Design review of the part built by this model. Coordinates are the model's own, in mm. Round coordinates to 2 decimals unless told otherwise and drop trailing zeros. Order: outer loops, then holes, each group sorted by start corner. A loop starts at its lowest first (then second) coordinate and runs counter-clockwise, first axis right, second up. Notation, with made-up numbers: M -17,42 L -13,42 A30 cw -13,67 Z; hole C -36.5,46 d1. An arc over 180 degrees is marked long. Write each question's results on one line, items separated by ' | '. Start each with the question number.
Item 1: Clearance check with a flat-ended pin moving along its axis: pin 1 (2 mm diameter, centred on x = 0, z = 0.5, fed in from -Y). State where the tip first meets the part, or that it passes through.
Item 2: Take a section at B-B, the plane y = 3.75. Write out the cut boundary in (x, z), plus the area to 3 significant figures.
Item 3: Take a section at A-A, the plane x = 0. Write out the cut boundary in (y, z).
Item 4: Take a section at C-C, the plane y = 2.25. Write out the cut boundary in (x, z), plus the area to 3 significant figures.
Item 5: Wall thickness on line 1 (Z direction, x = 0, y = 0.3); line 2 (X direction, y = 0.5, z = 0.25); line 3 (Z direction, x = 0.75, y = 2.5): over which ranges is each line inside the solid? List them lowest first. Write a range as [from, to].
Item 6: The part is to be moulded in two halves that separate along Z. For faces 1 (the flat face through (0, 0, 0.4)), 2 (the conical face through (1.198, 5.07, -0.377)), 3 (the flat face through (0.01, 1, 0.45)), say which applies: +Z half, -Z half, draft (parallel to the pull), parting line (faces both ways), or undercut.
```python
from build123d import *

# Parameters (mm, degrees)
IZIM1_R                     = 1.7
Y_KSEKLIK_EKSTR_ZYON1_DEPTH = 10
Y_KSEKLIK_EKSTR_ZYON1_TAPER = 5
IZIM2_R                     = 1.122825905
KES_EKSTR_ZYON1_DEPTH       = 10
KES_EKSTR_ZYON1_TAPER       = 4
IZIM3_R                     = 1.122825905
IZIM3_R_2                   = 0.19962026
IZIM3_R_3                   = 0.196792851
IZIM3_R_4                   = 0.203205658
IZIM3_R_5                   = 0.197119951
Y_KSEKLIK_EKSTR_ZYON3_DEPTH = 1
IZIM5_R                     = 0.197735833
IZIM5_R_2                   = 0.2
KES_EKSTR_ZYON2_DEPTH       = 1
IZIM6_R                     = 0.196695493
KES_EKSTR_ZYON3_DEPTH       = 1


with BuildPart() as part:
    # Çizim1 → Yükseklik-Ekstrüzyon1 (new body)
    with BuildSketch(Plane(origin=(0, 0, 0), x_dir=(1, 0, 0), z_dir=(0, 1, 0))):
        Circle(IZIM1_R)
    extrude(amount=Y_KSEKLIK_EKSTR_ZYON1_DEPTH, taper=Y_KSEKLIK_EKSTR_ZYON1_TAPER)

    # Çizim2 → Kes-Ekstrüzyon1 (cut)
    with BuildSketch(Plane.XZ):
        Circle(IZIM2_R)
    extrude(amount=-KES_EKSTR_ZYON1_DEPTH, taper=KES_EKSTR_ZYON1_TAPER, mode=Mode.SUBTRACT)

    # Çizim3 → Yükseklik-Ekstrüzyon3 (add)
    with BuildSketch(Plane(origin=(0, 0, 0), x_dir=(-1, 0, 0), z_dir=(0, -1, 0))):
        Circle(IZIM3_R)
        with Locations((-0.353553391, -0.353553391)):
            Circle(IZIM3_R_2, mode=Mode.SUBTRACT)
        with Locations((-0.353553391, 0.353553391)):
            Circle(IZIM3_R_3, mode=Mode.SUBTRACT)
        with Locations((0.353553391, 0.353553391)):
            Circle(IZIM3_R_4, mode=Mode.SUBTRACT)
        with Locations((0.353553391, -0.353553391)):
            Circle(IZIM3_R_5, mode=Mode.SUBTRACT)
    extrude(amount=-Y_KSEKLIK_EKSTR_ZYON3_DEPTH)

    # Çizim5 → Kes-Ekstrüzyon2 (cut)
    with BuildSketch(Plane.XZ):
        with Locations((0.8, 0)):
            Circle(IZIM5_R)
        with Locations((-0.8, 0)):
            Circle(IZIM5_R_2)
        with Locations((0, -0.8)):
            Circle(IZIM5_R)
        with Locations((0, 0.8)):
            Circle(IZIM5_R_2)
    extrude(amount=-KES_EKSTR_ZYON2_DEPTH, mode=Mode.SUBTRACT)

    # Çizim6 → Kes-Ekstrüzyon3 (cut)
    with BuildSketch(Plane.XZ):
        Circle(IZIM6_R)
    extrude(amount=-KES_EKSTR_ZYON3_DEPTH, mode=Mode.SUBTRACT)


solid = part.part
```
Results list:
1) pin 1: y = 0
2) outline: C 0,0 d2.74; hole C 0,0 d1.72 | area: 3.59 mm²
3) outline: M 0,-1.7 L 10,-0.83 L 10,-0.42 L 1,-1.05 L 1,-1 L 0,-1 Z; M 0,-0.6 L 1,-0.6 L 1,-0.2 L 0,-0.2 Z; M 0,0.2 L 1,0.2 L 1,0.6 L 0,0.6 Z; M 0,1 L 1,1 L 1,1.05 L 10,0.42 L 10,0.83 L 0,1.7 Z
4) outline: C 0,0 d3.01; hole C 0,0 d1.93 | area: 4.17 mm²
5) line 1: [-1.67, -1], [-0.6, -0.2], [0.2, 0.6], [1, 1.67] | line 2: [-1.64, -0.52], [-0.19, 0.18], [0.52, 1.64] | line 3: [-1.28, -0.58], [0.58, 1.28]
6) face 1: draft | face 2: parting line | face 3: undercut
